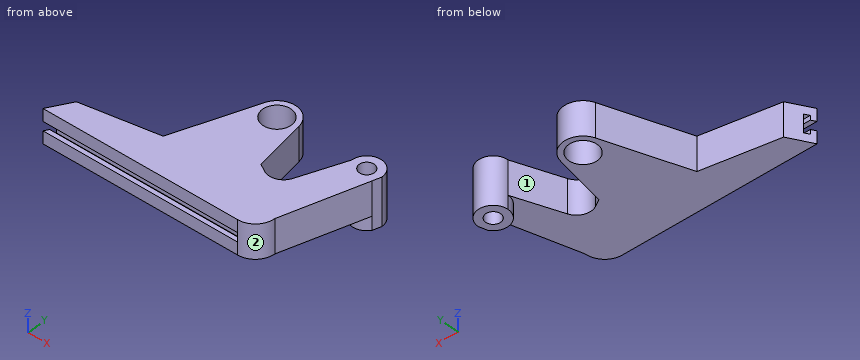
```python
from build123d import *

# Parameters (mm, degrees)
SKETCH1_R           = 13
SKETCH1_R_2         = 9.5
SKETCH1_R_3         = 5
BOSS_EXTRUDE1_DEPTH = 22.5
SKETCH6_W           = 3
SKETCH6_H           = 3
CUT_EXTRUDE2_DEPTH  = 130
FILLET1_R           = 10
SKETCH7_R           = 5
BOSS_EXTRUDE2_DEPTH = 9


with BuildPart() as part:
    # Sketch1 → Boss-Extrude1 (new body)
    # profile 1 of 7: a face of its own
    with BuildSketch(Plane.XY):
        with BuildLine():
            ThreePointArc((103.274249999, 72.665631876), (88.01682369, 59.863131087), (78.058245929, 77.11189374))
            Line((78.058245929, 77.11189374), (58.660254038, 23.816349035))
            Line((58.660254038, 23.816349035), (8.660254038, 15))
            Line((8.660254038, 15), (0, 0))
            Line((0, 0), (130, 0))
            ThreePointArc((130, 0), (120.807611845, 3.807611845), (117, 13))
            ThreePointArc((117, 13), (117.888810571, 17.724308479), (120.433706247, 21.802614602))
            Line((120.433706247, 21.802614602), (124.168764572, 31.377772343))
            Line((124.168764572, 31.377772343), (109.234628196, 40))
            Line((109.234628196, 40), (103.076750789, 74.923058186))
            ThreePointArc((103.076750789, 74.923058186), (103.224781075, 73.798656532), (103.274249999, 72.665631876))
        make_face()
    # profile 2 of 7: a face of its own
    with BuildSketch(Plane.XY):
        with Locations((90.274249999, 72.665631876)):
            Circle(SKETCH1_R)
        with Locations(Location((90.274249999, 72.665631876, 0), (0, 0, 180))):
            Circle(SKETCH1_R_2, mode=Mode.SUBTRACT)
    # profile 3 of 7: a face of its own
    with BuildSketch(Plane.XY):
        with BuildLine():
            Line((136.5, 24.258330249), (124.168764572, 31.377772343))
            Line((124.168764572, 31.377772343), (120.433706247, 21.802614602))
            ThreePointArc((120.433706247, 21.802614602), (128.035776443, 25.850751955), (136.5, 24.258330249))
        make_face()
    # profile 4 of 7: a face of its own
    with BuildSketch(Plane.XY):
        with BuildLine():
            ThreePointArc((117, 13), (120.807611845, 3.807611845), (130, 0))
            ThreePointArc((130, 0), (139.192388155, 3.807611845), (143, 13))
            ThreePointArc((143, 13), (141.258330249, 19.5), (136.5, 24.258330249))
            ThreePointArc((136.5, 24.258330249), (128.035776443, 25.850751955), (120.433706247, 21.802614602))
            Line((120.433706247, 21.802614602), (117, 13))
        make_face()
    # profile 5 of 7: a face of its own
    with BuildSketch(Plane.XY):
        with BuildLine():
            Line((117, 13), (120.433706247, 21.802614602))
            ThreePointArc((120.433706247, 21.802614602), (117.888810571, 17.724308479), (117, 13))
        make_face()
    # profile 6 of 7: a face of its own
    with BuildSketch(Plane.XY):
        with BuildLine():
            Line((140.274249999, 72.665631876), (124.168764572, 31.377772343))
            Line((124.168764572, 31.377772343), (136.5, 24.258330249))
            ThreePointArc((136.5, 24.258330249), (141.258330249, 19.5), (143, 13))
            Line((143, 13), (158.72749128, 67.323093917))
            ThreePointArc((158.72749128, 67.323093917), (147.493280097, 63.060101886), (140.274249999, 72.665631876))
        make_face()
    # profile 7 of 7: a face of its own
    with BuildSketch(Plane.XY):
        with BuildLine():
            ThreePointArc((160.274249999, 72.665631876), (150.274249999, 82.665631876), (140.274249999, 72.665631876))
            ThreePointArc((140.274249999, 72.665631876), (147.493280097, 63.060101886), (158.72749128, 67.323093917))
            Line((158.72749128, 67.323093917), (160.274249999, 72.665631876))
        make_face()
        with Locations(Location((150.274249999, 72.665631876, 0), (0, 0, 180))):
            Circle(SKETCH1_R_3, mode=Mode.SUBTRACT)
    extrude(amount=BOSS_EXTRUDE1_DEPTH)

    # Sketch6 → Cut-Extrude2 (cut)
    with BuildSketch(Plane(origin=(0, 0, 0), x_dir=(0, 0, -1), z_dir=(-1, 0, 0))):
        with Locations((-9.75, -1.5)):
            Rectangle(SKETCH6_W, SKETCH6_H)
        Polygon((-8.25, -3), (-11.25, -3), (-11.25, -6), (-5.25, -6), (-5.25, -3), align=None)
        with Locations((-12.75, -1.5)):
            Rectangle(SKETCH6_W, SKETCH6_H)
        Polygon((-11.25, -3), (-14.25, -3), (-17.25, -3), (-17.25, -6), (-11.25, -6), align=None)
    extrude(amount=-CUT_EXTRUDE2_DEPTH, mode=Mode.SUBTRACT)

    # Fillet1
    fillet1_edges = [part.edges().sort_by_distance(p)[0] for p in [
        (124.168764572, 31.377772343, 11.25),
    ]]
    fillet(fillet1_edges, radius=FILLET1_R)

    # Sketch7 → Boss-Extrude2 (add)
    with BuildSketch(Plane.XY.offset(22.5)):
        with BuildLine():
            Line((158.72749128, 67.323093917), (160.274249999, 72.665631876))
            ThreePointArc((160.274249999, 72.665631876), (150.274249999, 82.665631876), (140.274249999, 72.665631876))
            ThreePointArc((140.274249999, 72.665631876), (147.493280097, 63.060101886), (158.72749128, 67.323093917))
        make_face()
        with Locations(Location((150.274249999, 72.665631876, 0), (0, 0, 180))):
            Circle(SKETCH7_R, mode=Mode.SUBTRACT)
    extrude(amount=BOSS_EXTRUDE2_DEPTH)


with BuildPart() as body_2:
    # Mirror1: mirrored copy
    add(part.part.mirror(Plane.XY))


solid = body_2.part
```
For this review, take the finished solid that the model builds, in its own axes (mm). Face numbers are marked on the shaded views. A direction names the side the tool comes from. Give positions to 0.01 mm unless a question says otherwise; leave off trailing zeros. Write each loop counter-clockwise with the first axis right and the second up, starting at its lowest first coordinate (ties: lowest second). Pieces come first, ordered by that corner, then holes.
Item 1: Wall thickness on probe 1 along Z at (x, y) = (47, 5); probe 2 along Z at (x, y) = (65, 40.5); probe 3 along X at (y, z) = (76.5, -9): over which ranges is each line inside the solid? List them lowest first.
Item 2: Machinability: for the marked faces 1 and 2, which of the approach directions +Z, -Z, +X, -X, +Y, -Y give a long, thin tool a straight path to every point of the face, cutting with its end or side? Answer none if there is none.
Item 3: Take a section at A-A (z = -2). Give the boundary of the cut face in (x, y), and give its area (3 significant figures).
Item 4: Take a section at D-D (x = 74.5). Give the boundary of the cut face in (y, z).
Item 5: Insertion check: P1, Ø3.5, axis at x = 34.5, y = 4.5, coming from the -Z side; P2, Ø2.5, axis at x = 97.5, z = -15, coming from the +Y side; P3, Ø4, axis at y = 34.5, z = -8, coming from the -X side. Each pin has a flat end and moves straight along its axis. Give the tip position at first contact, or say it passes through.
Item 6: Take a section at C-C (x = 149). Give the boundary of the cut face in (y, z), and give its area (3 significant figures).
Item 7: Take a section at B-B (y = 49.5). Give the boundary of the cut face in (x, z).
Established:
1. probe 1: z = -22.5 to -17.25, -5.25 to 0
1. probe 2: z = -22.5 to 0
1. probe 3: x = 77.84 to 81.58, 98.97 to 102.7, 141.04 to 147.07, 153.48 to 159.51
2. face 1: +Z, -Z, +Y
2. face 2: +Z, -Z, +X, -Y
3. outline: (0, 0) - (130, 0) arc R13 ccw to (143, 13) - (160.27, 72.67) arc R10 ccw to (140.27, 72.67) - (128.4, 42.23) arc R10 cw to (114.08, 37.2) - (109.23, 40) - (103.08, 74.92) arc R13 ccw to (78.06, 77.11) - (58.66, 23.82) - (8.66, 15) - close; hole circle Ø19 at (90.27, 72.67); hole circle Ø10 at (150.27, 72.67)
3. area: 6,320 mm2
4. outline: (0, -22.5) - (67.34, -22.5) - (67.34, 0) - (0, 0) - (0, -8.25) - (3, -8.25) - (3, -5.25) - (6, -5.25) - (6, -17.25) - (3, -17.25) - (3, -14.25) - (0, -14.25) - close
5. P1: stops at z = -22.5
5. P2: stops at y = 84.21
5. P3: stops at x = 61.82
6. outline: (33.72, -22.5) - (62.75, -22.5) - (62.75, -31.5) - (67.83, -31.5) - (67.83, 0) - (33.72, 0) - close; (77.5, -31.5) - (82.58, -31.5) - (82.58, 0) - (77.5, 0) - close
6. area: 973 mm2
7. outline: (68.01, -22.5) - (107.56, -22.5) - (107.56, 0) - (68.01, 0) - close; (131.24, -22.5) - (153.57, -22.5) - (153.57, 0) - (131.24, 0) - close
